Here's how the part is built. I have some questions about the finished solid (model axes, mm). Round coordinates to 2 decimals unless told otherwise and drop trailing zeros. Write each loop counter-clockwise with the first axis right and the second up, starting at its lowest first coordinate (ties: lowest second). Pieces come first, ordered by that corner, then holes. Notation, with made-up numbers: (75.25, 10) -> (101.25, 10) arc R21 cw to (101.25, 19) -> close; hole circle Ø9 at (-17.5, 81). An arc over 180 degrees is marked (long way). Answer in a Markdown table with one row per item. Add a question column.
from build123d import *

# Parameters (mm, degrees)
F0_R     = 11
F1_DEPTH = 1.2
F2_R     = 1
F3_R     = 1.55
F3_R_2   = 3.4
F4_DEPTH = 25


with BuildPart() as f1:
    # F0 (on Top) → F1 (new body)
    with BuildSketch(Plane.XY):
        Circle(F0_R)
    extrude(amount=F1_DEPTH)

    # F2
    f2_edges = [f1.edges().sort_by_distance(p)[0] for p in [
        (-11, 0, 1.2),
    ]]
    fillet(f2_edges, radius=F2_R)

    # F3 (on face) → F4 (cut)
    with BuildSketch(Plane.XY.offset(1.2)):
        Circle(F3_R)
        with Locations((0, 7)):
            Circle(F3_R_2)
    extrude(amount=-F4_DEPTH, mode=Mode.SUBTRACT)


solid = f1.part
Item 1: If we mould it in two halves opening along X, with no side actions, what happens to faces 1 (the cylindrical face through (0.715, -1.375, 0.608)), 2 (the flat face through (0, -2, 0))? For each: pulls with the +X half, pulls with the -X half, needs draft (parallel to the pull), parting line crosses it, or undercut.
Item 2: If we section it at C-C on x = 0: Please give me the cut outline in (y, z).
Item 3: I need wall thicknesses on line 1 along Y through (x, z) = (0, 0.35); line 2 along Y through (x, z) = (0, 0.95); line 3 along X through (y, z) = (7, 0.6). Which ranges of each line are inside material? Lowest first, please. Write a range as from..to.
Item 4: If we section it at A-A on y = 0: Please give me the cut outline in (x, z), then the cut area to 3 significant figures.
Item 5: If we section it at B-B on z = 0.8: Please give me the cut outline in (x, y), then the cut area to 3 significant figures.
Results list:
| question | item | result |
|---|---|---|
| 1 | face 1 | undercut |
| 1 | face 2 | needs draft |
| 2 | outline | (-11, 0) -> (-1.55, 0) -> (-1.55, 1.2) -> (-10, 1.2) arc R1 ccw to (-11, 0.2) -> close; (1.55, 0) -> (3.6, 0) -> (3.6, 1.2) -> (1.55, 1.2) -> close; (10.4, 0) -> (11, 0) -> (11, 0.2) arc R1 ccw to (10.4, 1.12) -> close |
| 3 | line 1 | -10.99..-1.55, 1.55..3.6, 10.4..10.99 |
| 3 | line 2 | -10.66..-1.55, 1.55..3.6, 10.4..10.66 |
| 3 | line 3 | -8.38..-3.4, 3.4..8.38 |
| 4 | outline | (-11, 0) -> (-1.55, 0) -> (-1.55, 1.2) -> (-10, 1.2) arc R1 ccw to (-11, 0.2) -> close; (1.55, 0) -> (11, 0) -> (11, 0.2) arc R1 ccw to (10, 1.2) -> (1.55, 1.2) -> close |
| 4 | area | 22.3 mm² |
| 5 | outline | circle Ø21.6 at (0, 0); hole circle Ø6.8 at (0, 7); hole circle Ø3.1 at (0, 0) |
| 5 | area | 323 mm² |
